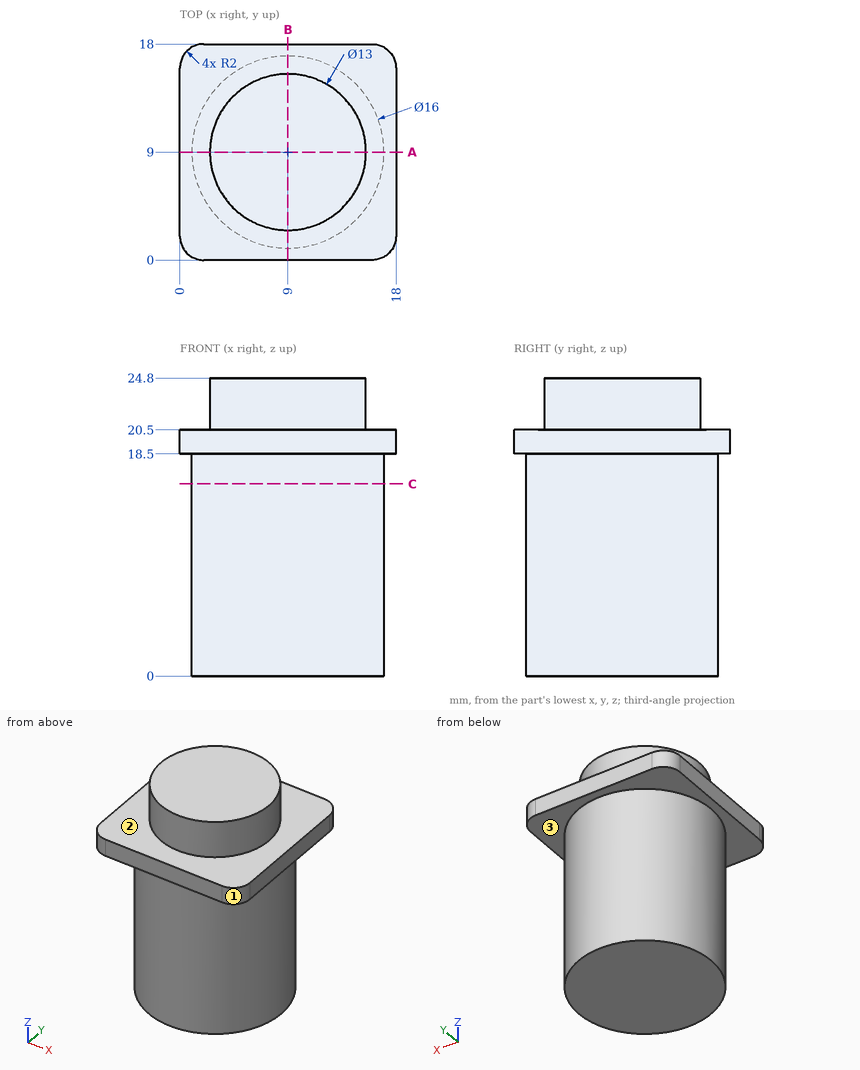
Source: three-view drawing plus pictorial views. Frame: mm from the lowest corner of the part. A direction names the side the tool comes from. Coordinates: 2 decimals unless noted, no trailing zeros. Loops run counter-clockwise (first coordinate to the right, second up) from the corner with the lowest first, then second, coordinate; pieces in that order, holes last. Notation, with made-up numbers: (-16.5, 4) -> (34.5, 4) arc R29 ccw to (34.5, 31) -> close; hole circle Ø9 at (-8, 51). An arc over 180 degrees is marked (long way). Write each question's results on one line, items separated by ' | '. Start each with the question number.
Q1. Section A-A, the plane y = 9. Return the cut outline in (x, z).
Q2. Pin query (flat end, axial travel): pin 1 (6 mm diameter, centred on y = 11.5, z = 5, fed in from -X); pin 2 (10 mm diameter, centred on x = 3, z = 13, fed in from -Y); pin 3 (10 mm diameter, centred on y = 9, z = 9, fed in from +X). Return the tip coordinate at first contact, or that it passes through.
Q3. Reachability of the marked faces 1, 2 and 3 from +Z, -Z, +X, -X, +Y, -Y: full face, straight path, thin tool, end or side. Return the list, or none.
Q4. Section C-C, the plane z = 16. Return the cut outline in (x, y), plus the area to 3 significant figures.
Q5. Ray query, line 1 (Z direction, x = 16, y = 9.5); line 2 (Z direction, x = 16.25, y = 2.75); line 3 (Y direction, x = 7.25, z = 8.75). Return the intervals inside material, ascending. Write a range as from..to.
Found:
1) outline: (0, 18.5) -> (1, 18.5) -> (1, 0) -> (17, 0) -> (17, 18.5) -> (18, 18.5) -> (18, 20.5) -> (15.5, 20.5) -> (15.5, 24.8) -> (2.5, 24.8) -> (2.5, 20.5) -> (0, 20.5) -> close
2) pin 1: x = 1 | pin 2: y = 1.06 | pin 3: x = 17
3) face 1: +Z, -Z, +X, -Y | face 2: +Z | face 3: -Z
4) outline: circle Ø16 at (9, 9) | area: 201 mm2
5) line 1: 0..20.5 | line 2: 18.5..20.5 | line 3: 1.19..16.81
